from build123d import *

# Parameters (mm, degrees)
SKETCH1_R           = 1.5
BOSS_EXTRUDE1_DEPTH = 1


with BuildPart() as part:
    # Sketch1 → Boss-Extrude1 (new body)
    with BuildSketch(Plane.XY):
        with BuildLine():
            Line((-13.546388506, 1.11267473), (-14.757525988, -4.995272772))
            ThreePointArc((-14.757525988, -4.995272772), (-16.032025568, -6.905175586), (-18.283738095, -7.354473522))
            Line((-18.283738095, -7.354473522), (-19.594124086, -7.094638677))
            ThreePointArc((-19.594124086, -7.094638677), (-20.344694929, -7.244404656), (-20.769528122, -7.881038927))
            Line((-20.769528122, -7.881038927), (-21.639356034, -12.267711208))
            ThreePointArc((-21.639356034, -12.267711208), (-21.489590055, -13.018282051), (-20.852955784, -13.443115244))
            Line((-20.852955784, -13.443115244), (-11.13347013, -15.370380234))
            ThreePointArc((-11.13347013, -15.370380234), (-8.873016287, -14.915211716), (-7.60323447, -12.990508078))
            Line((-7.60323447, -12.990508078), (-6.569563046, -7.578700869))
            ThreePointArc((-6.569563046, -7.578700869), (-0.732388238, 4.25291316), (-13.546388506, 1.11267473))
        make_face()
        with Locations((-12.024833612, -12.026666232)):
            Circle(SKETCH1_R, mode=Mode.SUBTRACT)
    extrude(amount=BOSS_EXTRUDE1_DEPTH)


solid = part.part
Check sheet for the modelled part. Datum: model origin and axes. Units: mm. A direction names the side the tool comes from. Give positions to 0.01 mm unless a question says otherwise; leave off trailing zeros. Write each loop counter-clockwise with the first axis right and the second up, starting at its lowest first coordinate (ties: lowest second). Pieces come first, ordered by that corner, then holes. Notation, with made-up numbers: (23.25, -37) -> (55.25, -37) arc R18 ccw to (55.25, -16) -> close; hole circle Ø2 at (-1, -39). An arc over 180 degrees is marked (long way). One line per item, written item: value. Start each with the question number.
Item 1: Material ranges on probe 1 along Y at (x, z) = (-11.25, 0.1); probe 2 along Y at (x, z) = (-12.5, 0.6); probe 3 along X at (y, z) = (1.75, 0.6), recorded low to high. Write a range as from..to.
Item 2: Section check A-A on z = 0.8. Record the cut outline in (x, y).
Item 3: Section check C-C on x = -9.75. Record the cut outline in (y, z).
Item 4: Draft check along X on faces 3 (the cylindrical face through (-21.5, -13, 0.5)), 4 (the cylindrical face through (-11.22, -10.76, 0.49)), 5 (the cylindrical face through (-0.59, 4.07, 0.49)). Enter one of: +X half, -X half, draft (parallel to the pull), parting line (faces both ways), or undercut.
Item 5: Section check D-D on y = -8.5. Record the cut outline in (x, z), then the cut area to 3 significant figures.
Item 6: Section check B-B on x = -13. Record the cut outline in (y, z).
Item 7: Tool access check on faces 1 (the flat face through (-21.198, -10.044, 0.493)), 2 (the flat face through (-18.93, -7.226, 0.493)). Record the directions out of +Z, -Z, +X, -X, +Y, -Y that give a thin tool (end or side, any length) a straight path to the whole face; none if there is none.
Results list:
1. probe 1: -15.35..-13.31, -10.74..5.13
1. probe 2: -15.1..-13.45, -10.6..3.68
1. probe 3: -13.39..0.57
2. outline: (-21.64, -12.27) arc R1 ccw to (-20.85, -13.44) -> (-11.13, -15.37) arc R3 ccw to (-7.6, -12.99) -> (-6.57, -7.58) arc R7.28 ccw (long way) to (-13.55, 1.11) -> (-14.76, -5) arc R3 cw to (-18.28, -7.35) -> (-19.59, -7.09) arc R1 ccw to (-20.77, -7.88) -> close; hole circle Ø3 at (-12.02, -12.03)
3. outline: (-15.32, 0) -> (6.16, 0) -> (6.16, 1) -> (-15.32, 1) -> close
4. face 3: -X half
4. face 4: undercut
4. face 5: parting line
5. outline: (-20.89, 0) -> (-6.75, 0) -> (-6.75, 1) -> (-20.89, 1) -> close
5. area: 14.1 mm²
6. outline: (-15, 0) -> (-13.17, 0) -> (-13.17, 1) -> (-15, 1) -> close; (-10.89, 0) -> (2.78, 0) -> (2.78, 1) -> (-10.89, 1) -> close
7. face 1: +Z, -Z, -X, +Y
7. face 2: +Z, -Z, +Y
